```python
from build123d import *

# Parameters (mm, degrees)
BOX_W           = 70
BOX_H           = 42
BOX_DEPTH       = 17
SKETCH_R        = 1.75
POCKET_DEPTH    = 70.001
POCKET001_DEPTH = 50
POCKET002_DEPTH = 35
SKETCH003_R     = 6.75
POCKET003_DEPTH = 17.001
SKETCH004_R     = 8.25
POCKET004_DEPTH = 8.3
SKETCH005_R     = 8.25
POCKET005_DEPTH = 4.2


with BuildPart() as part:
    # Box → Box (new body)
    with BuildSketch(Plane.XY):
        with Locations((35, 21)):
            Rectangle(BOX_W, BOX_H)
    extrude(amount=BOX_DEPTH)

    # Sketch (on Face2 of BaseFeature) → Pocket (cut, through all)
    with BuildSketch(Plane.YZ.offset(70)):
        with Locations((5.5, 13.25)):
            Circle(SKETCH_R)
        with Locations((36.5, 13.25)):
            Circle(SKETCH_R)
    extrude(amount=-POCKET_DEPTH, mode=Mode.SUBTRACT)

    # Sketch001 (on Face2 of BaseFeature) → Pocket001 (cut)
    with BuildSketch(Plane.YZ.offset(70)):
        Polygon((4, 17), (0, 17), (0, 13), align=None)
        Polygon((38, 17), (42, 17), (42, 13), align=None)
    extrude(amount=-POCKET001_DEPTH, mode=Mode.SUBTRACT)

    # Sketch002 (on Face8 of Pocket001) → Pocket002 (cut)
    with BuildSketch(Plane.YZ.offset(70)):
        Polygon((4, 17), (0, 13), (0, 10.5), (3.5, 7), (38.5, 7), (42, 10.5), (42, 13), (38, 17), align=None)
    extrude(amount=-POCKET002_DEPTH, mode=Mode.SUBTRACT)

    # Sketch003 (on Face3 of Pocket002) → Pocket003 (cut, through all)
    with BuildSketch(Plane.XY.offset(17)):
        with Locations((27, 27)):
            Circle(SKETCH003_R)
    extrude(amount=-POCKET003_DEPTH, mode=Mode.SUBTRACT)

    # Sketch004 (on Face3 of Pocket003) → Pocket004 (cut)
    with BuildSketch(Plane.XY.offset(17)):
        with Locations((27, 27)):
            Circle(SKETCH004_R)
    extrude(amount=-POCKET004_DEPTH, mode=Mode.SUBTRACT)

    # Sketch005 (on Face4 of Pocket004) → Pocket005 (cut)
    with BuildSketch(Plane(origin=(0, 0, 0), x_dir=(1, 0, 0), z_dir=(0, 0, -1))):
        with Locations((27, -27)):
            Circle(SKETCH005_R)
    extrude(amount=-POCKET005_DEPTH, mode=Mode.SUBTRACT)


solid = part.part
```
The model under review builds one solid part; all positions refer to its coordinate system, in mm. A direction names the side the tool comes from. Round coordinates to 2 decimals unless told otherwise and drop trailing zeros. Loops run counter-clockwise (first coordinate to the right, second up) from the corner with the lowest first, then second, coordinate; pieces in that order, holes last. Notation, with made-up numbers: (-37, 32.5) -> (-28, 32.5) arc R24 ccw to (-28, 53.5) -> close; hole circle Ø8 at (-26, -31). An arc over 180 degrees is marked (long way). Answer in a Markdown table with one row per item.
1) Consider section B-B, the plane x = 24.5. Write out the cut boundary in (y, z).
Taken from the geometry:
| item | result |
|---|---|
| outline | (0, 0) -> (19.14, 0) -> (19.14, 4.2) -> (20.73, 4.2) -> (20.73, 8.7) -> (19.14, 8.7) -> (19.14, 17) -> (4, 17) -> (0, 13) -> close; (33.27, 4.2) -> (34.86, 4.2) -> (34.86, 0) -> (42, 0) -> (42, 13) -> (38, 17) -> (34.86, 17) -> (34.86, 13.87) arc R1.75 cw (long way) to (34.86, 12.63) -> (34.86, 8.7) -> (33.27, 8.7) -> close; hole circle Ø3.5 at (5.5, 13.25) |
2) Consider section D-D, the plane y = 5.5. Write out the cut boundary in (x, z), plus the area to 4 significant figures.
Taken from the geometry:
| item | result |
|---|---|
| outline | (0, 0) -> (70, 0) -> (70, 7) -> (35, 7) -> (35, 11.5) -> (0, 11.5) -> close; (0, 15) -> (35, 15) -> (35, 17) -> (0, 17) -> close |
| area | 717.5 mm² |
3) Wall thickness on line 1 along Y through (x, z) = (27, 3.2); line 2 along Y through (x, z) = (27, 12.75); line 3 along Z through (x, y) = (10, 36.5): over which ranges is each line inside the solid? List them lowest first.
Taken from the geometry:
| item | result |
|---|---|
| line 1 | y = 0 to 18.75, 35.25 to 42 |
| line 2 | y = 0 to 3.82, 7.18 to 18.75, 38.18 to 42 |
| line 3 | z = 0 to 11.5, 15 to 17 |
4) Tool access review of faces 1 (the flat face through (35, 21, 12)), 2 (the flat face through (20, 1.5, 15.5)), 3 (the flat face through (0, 21, 8)), 4 (the flat face through (28, 40, 15)), 5 (the cylindrical face through (20.453, 32.02, 2.071)): name each direction out of +Z, -Z, +X, -X, +Y, -Y from which nothing blocks a thin tool from reaching the whole face with its end or side.
Taken from the geometry:
| item | result |
|---|---|
| face 1 | +Z, +X |
| face 2 | +Z, +X, -Y |
| face 3 | +Z, -Z, -X, +Y, -Y |
| face 4 | +Z, +X, +Y |
| face 5 | -Z |
5) Consider section C-C, the plane z = 1.5. Write out the cut boundary in (x, y).
Taken from the geometry:
| item | result |
|---|---|
| outline | (0, 0) -> (70, 0) -> (70, 42) -> (0, 42) -> close; hole circle Ø16.5 at (27, 27) |
6) Consider section A-A, the plane y = 27. Write out the cut boundary in (x, z).
Taken from the geometry:
| item | result |
|---|---|
| outline | (0, 0) -> (18.75, 0) -> (18.75, 4.2) -> (20.25, 4.2) -> (20.25, 8.7) -> (18.75, 8.7) -> (18.75, 17) -> (0, 17) -> close; (33.75, 4.2) -> (35.25, 4.2) -> (35.25, 0) -> (70, 0) -> (70, 7) -> (35, 7) -> (35, 8.7) -> (33.75, 8.7) -> close |
7) Draft analysis for pull direction X (two halves, no side actions). For faces 6 (the flat face through (35, 42, 6)), 7 (the flat face through (20, 40.5, 15.5)), 8 (the cylindrical face through (22.025, 31.562, 6.481)), state which applies: pulls with the +X half, pulls with the -X half, needs draft (parallel to the pull), parting line crosses it, or undercut.
Taken from the geometry:
| item | result |
|---|---|
| face 6 | needs draft |
| face 7 | pulls with the +X half |
| face 8 | undercut |
8) For pin 1 Ø3 at (y, z) = (5.5, 13.25) entering from +X; pin 2 Ø2 at (y, z) = (2.5, 14) entering from +X; pin 3 Ø15 at (x, y) = (27, 27) entering from -Z; pin 4 Ø13 at (x, y) = (28, 27.5) entering from +Z, all flat-tipped, find the tip position at first contact; note any pin that passes through.
Taken from the geometry:
| item | result |
|---|---|
| pin 1 | passes through |
| pin 2 | stops at x = 35 |
| pin 3 | stops at z = 4.2 |
| pin 4 | stops at z = 8.7 |
